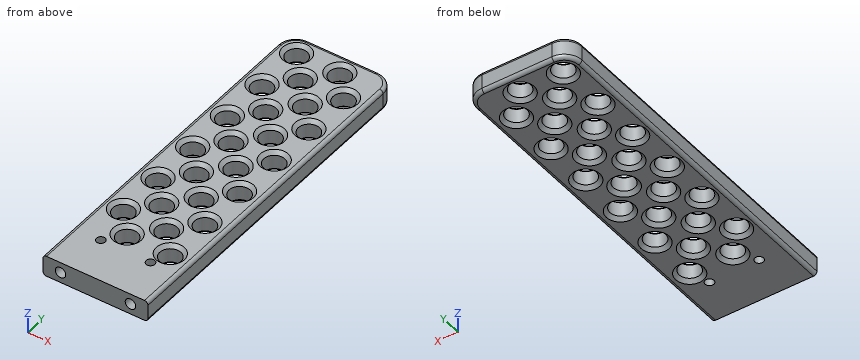
```python
from build123d import *

# Parameters (mm, degrees)
F0_W     = 30
F0_H     = 100
F0_R     = 1.25
F1_DEPTH = 6
F2_R     = 3
F2_R_2   = 3.0525598616
F3_DEPTH = 6.001
F4_R     = 5
F5_SIZE  = 1
F6_R     = 1
F7_R     = 1.5
F8_DEPTH = 6


with BuildPart() as f1:
    # F0 (on Top) → F1 (new body)
    with BuildSketch(Plane.XY):
        Rectangle(F0_W, F0_H)
        with Locations((-7.1, -37.8)):
            Circle(F0_R, mode=Mode.SUBTRACT)
        with Locations((7.1, -37.8)):
            Circle(F0_R, mode=Mode.SUBTRACT)
    extrude(amount=F1_DEPTH)

    # F2 (on Top) → F3 (cut, through all)
    with BuildSketch(Plane.XY):
        with Locations((-9.3485760093, -25.5)):
            Circle(F2_R)
        with Locations((-3.3485760093, -18.5)):
            Circle(F2_R)
        with Locations((3, -25.5)):
            Circle(F2_R)
        with Locations((9, -18.5)):
            Circle(F2_R)
        with Locations((9, -32.5)):
            Circle(F2_R)
        with Locations((-3.3485760093, -32.4681438506)):
            Circle(F2_R)
        with Locations((-9.3485760093, -11.5)):
            Circle(F2_R)
        with Locations((3, -11.5)):
            Circle(F2_R)
        with Locations((-3.3485760093, -4.5)):
            Circle(F2_R)
        with Locations((3, 2.5)):
            Circle(F2_R_2)
        with Locations((9, 9.498416102)):
            Circle(F2_R)
        with Locations((-3.3485760093, 9.498416102)):
            Circle(F2_R)
        with Locations((-9.3485760093, 16.498416102)):
            Circle(F2_R)
        with Locations((3, 16.498416102)):
            Circle(F2_R)
        with Locations((-3.3485760093, 23.498416102)):
            Circle(F2_R)
        with Locations((-9.3485760093, 30.498416102)):
            Circle(F2_R)
        with Locations((3, 30.498416102)):
            Circle(F2_R)
        with Locations((-3.3485760093, 37.498416102)):
            Circle(F2_R)
        with Locations((-9.3485760093, 44.4896388961)):
            Circle(F2_R)
        with Locations((3, 44.4896388961)):
            Circle(F2_R)
        with Locations((9, -4.5)):
            Circle(F2_R)
        with Locations((9, 23.498416102)):
            Circle(F2_R)
        with Locations((9, 37.498416102)):
            Circle(F2_R)
        with Locations((-9.3485760093, 2.5)):
            Circle(F2_R)
    extrude(amount=F3_DEPTH, mode=Mode.SUBTRACT)

    # F4
    f4_edges = [f1.edges().sort_by_distance(p)[0] for p in [
        (15, 50, 3),
        (-15, 50, 3),
    ]]
    fillet(f4_edges, radius=F4_R)

    # F5
    f5_edges = [f1.edges().sort_by_distance(p)[0] for p in [
        (-6.348576, -32.468144, 6),
        (-12.348576, -25.5, 6),
        (-6.348576, -18.5, 6),
        (0, -25.5, 6),
        (6, -32.5, 6),
        (6, -18.5, 6),
        (0, -11.5, 6),
        (-12.348576, -11.5, 6),
        (-6.348576, -4.5, 6),
        (-12.348576, 2.5, 6),
        (-0.05256, 2.5, 6),
        (6, -4.5, 6),
        (6, 9.498416, 6),
        (-6.348576, 9.498416, 6),
        (-12.348576, 16.498416, 6),
        (-6.348576, 23.498416, 6),
        (0, 16.498416, 6),
        (6, 23.498416, 6),
        (0, 30.498416, 6),
        (6, 37.498416, 6),
        (0, 44.489639, 6),
        (-6.348576, 37.498416, 6),
        (-12.348576, 44.489639, 6),
        (-12.348576, 30.498416, 6),
        (6, -32.5, 0),
        (-6.348576, -32.468144, 0),
        (-12.348576, -25.5, 0),
        (0, -25.5, 0),
        (6, -18.5, 0),
        (-6.348576, -18.5, 0),
        (-12.348576, -11.5, 0),
        (0, -11.5, 0),
        (6, -4.5, 0),
        (-6.348576, -4.5, 0),
        (-0.05256, 2.5, 0),
        (-12.348576, 2.5, 0),
        (-6.348576, 9.498416, 0),
        (6, 9.498416, 0),
        (0, 16.498416, 0),
        (-12.348576, 16.498416, 0),
        (6, 23.498416, 0),
        (-6.348576, 23.498416, 0),
        (-12.348576, 30.498416, 0),
        (0, 30.498416, 0),
        (6, 37.498416, 0),
        (-6.348576, 37.498416, 0),
        (0, 44.489639, 0),
        (-12.348576, 44.489639, 0),
    ]]
    chamfer(f5_edges, length=F5_SIZE)

    # F6
    f6_edges = [f1.edges().sort_by_distance(p)[0] for p in [
        (15, -2.5, 6),
        (15, -2.5, 0),
        (13.535534, 48.535534, 0),
    ]]
    fillet(f6_edges, radius=F6_R)

    # F7 (on face) → F8 (cut)
    with BuildSketch(Plane.XZ.offset(50)):
        with Locations((-10, 3)):
            Circle(F7_R)
        with Locations((10, 3)):
            Circle(F7_R)
    extrude(amount=-F8_DEPTH, mode=Mode.SUBTRACT)


solid = f1.part
```
Could you check a few things on this model? Use its own coordinates, in mm. Round coordinates to 2 decimals unless told otherwise and drop trailing zeros. Loops run counter-clockwise (first coordinate to the right, second up) from the corner with the lowest first, then second, coordinate; pieces in that order, holes last. Notation, with made-up numbers: M -10.5,53.5 L 36.5,53.5 A30 cw 36.5,91.5 Z; hole C 31.5,88 d1. An arc over 180 degrees is marked long. Write item = value, one per line.
1. Will these pins go through, and if not, where does the flat tip stop? P1, Ø3.5, axis at x = 3, y = 2.5, coming from the -Z side; P2, Ø7, axis at x = 3, y = -25.5, coming from the +Z side; P3, Ø1.8, axis at x = 10, z = 3, coming from the -Y side; P4, Ø7, axis at x = -9.35, y = -11.5, coming from the -Z side.
Results below:
P1 = through
P2 = 5.5
P3 = -44
P4 = 0.5
2. I want a section at C-C, the plane y = -37.8. Write out the boundary of the cut face in (x, z).
Results below:
outline = M -15,1 A1 ccw -14,0 L -8.35,0 L -8.35,6 L -14,6 A1 ccw -15,5 Z; M -5.85,0 L 5.85,0 L 5.85,6 L -5.85,6 Z; M 8.35,0 L 14,0 A1 ccw 15,1 L 15,5 A1 ccw 14,6 L 8.35,6 Z
3. I need wall thicknesses on probe 1 along X at (y, z) = (-18.5, 3.6); probe 2 along X at (y, z) = (-11.5, 3.3); probe 3 along Z at (x, y) = (-10, -45.5). Which ranges of each line are inside material? Lowest first, please.
Results below:
probe_1 = -15 to -6.35, -0.35 to 6, 12 to 15
probe_2 = -15 to -12.35, -6.35 to 0, 6 to 15
probe_3 = 0 to 1.5, 4.5 to 6
4. I want a section at A-A, the plane y = 2.5. Write out the boundary of the cut face in (x, z), and give its area (3 significant figures).
Results below:
outline = M -15,1 A1 ccw -14,0 L -13.35,0 L -12.35,1 L -12.35,5 L -13.35,6 L -14,6 A1 ccw -15,5 Z; M -6.35,1 L -5.35,0 L -1.05,0 L -0.05,1 L -0.05,5 L -1.05,6 L -5.35,6 L -6.35,5 Z; M 6.05,1 L 7.05,0 L 14,0 A1 ccw 15,1 L 15,5 A1 ccw 14,6 L 7.05,6 L 6.05,5 Z
area = 103 mm²
5. I want a section at B-B, the plane y = -18.5. Write out the boundary of the cut face in (x, z), and give its area (3 significant figures).
Results below:
outline = M -15,1 A1 ccw -14,0 L -7.35,0 L -6.35,1 L -6.35,5 L -7.35,6 L -14,6 A1 ccw -15,5 Z; M -0.35,1 L 0.65,0 L 5,0 L 6,1 L 6,5 L 5,6 L 0.65,6 L -0.35,5 Z; M 12,1 L 13,0 L 14,0 A1 ccw 15,1 L 15,5 A1 ccw 14,6 L 13,6 L 12,5 Z
area = 103 mm²
